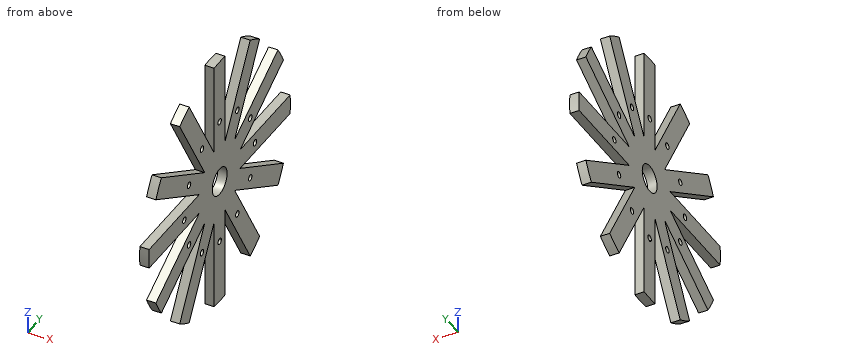
```python
from build123d import *

# Parameters (mm, degrees)
SKETCH1_W           = 450
SKETCH1_H           = 450
BOSS_EXTRUDE1_DEPTH = 5
BOSS_EXTRUDE2_DEPTH = 7.48
BOSS_EXTRUDE3_DEPTH = 7.48
SKETCH6_W           = 450
SKETCH6_H           = 450
CUT_EXTRUDE1_DEPTH  = 5
SKETCH7_R           = 11
SKETCH7_R_2         = 2.5
CUT_EXTRUDE2_DEPTH  = 10
SKETCH8_R           = 209.3091
SKETCH8_R_2         = 104.5891
CUT_EXTRUDE3_DEPTH  = 10
BOSS_EXTRUDE4_DEPTH = 7.48
SKETCH11_R          = 2.5
CUT_EXTRUDE5_DEPTH  = 10
SKETCH12_R          = 20.73675099
SKETCH12_R_2        = 11
BOSS_EXTRUDE5_DEPTH = 7.48


# Read off the part's stored shape, not the designer's step: Boss-Extrude2
with BuildPart() as part:
    # Sketch1 → Boss-Extrude1 (new body)
    with BuildSketch(Plane(origin=(0, 0, 0), x_dir=(0, 0, -1), z_dir=(1, 0, 0))):
        Rectangle(SKETCH1_W, SKETCH1_H)
    extrude(amount=BOSS_EXTRUDE1_DEPTH)

    # Boss-Extrude2 outline → Boss-Extrude2 (add)
    with BuildSketch(Plane(origin=(5, 0, 0), x_dir=(0, 0, -1), z_dir=(1, 0, 0))):
        with BuildLine():
            Line((-164.971757583, 8.09), (-209.152698388, 8.09))
            ThreePointArc((-209.152698388, 8.09), (-209.3091, 0), (-209.152698388, -8.09))
            Line((-209.152698388, -8.09), (-164.971757583, -8.09))
            ThreePointArc((-164.971757583, -8.09), (-116.792827049, -116.792827049), (-8.09, -164.971757583))
            Line((-8.09, -164.971757583), (-8.09, -209.152698388))
            ThreePointArc((-8.09, -209.152698388), (0, -209.3091), (8.09, -209.152698388))
            Line((8.09, -209.152698388), (8.09, -164.971757583))
            ThreePointArc((8.09, -164.971757583), (116.792827049, -116.792827049), (164.971757583, -8.09))
            Line((164.971757583, -8.09), (209.152698388, -8.09))
            ThreePointArc((209.152698388, -8.09), (209.3091, 0), (209.152698388, 8.09))
            Line((209.152698388, 8.09), (164.971757583, 8.09))
            ThreePointArc((164.971757583, 8.09), (116.792827049, 116.792827049), (8.09, 164.971757583))
            Line((8.09, 164.971757583), (8.09, 209.152698388))
            ThreePointArc((8.09, 209.152698388), (0, 209.3091), (-8.09, 209.152698388))
            Line((-8.09, 209.152698388), (-8.09, 164.971757583))
            ThreePointArc((-8.09, 164.971757583), (-116.792827049, 116.792827049), (-164.971757583, 8.09))
        make_face()
        with BuildLine():
            Line((148.770198629, 8.09), (104.538333308, 8.09))
            ThreePointArc((104.538333308, 8.09), (104.8509, 0), (104.538333308, -8.09))
            Line((104.538333308, -8.09), (148.770198629, -8.09))
            ThreePointArc((148.770198629, -8.09), (105.351839329, -105.351839329), (8.09, -148.770198629))
            Line((8.09, -148.770198629), (8.09, -104.538333308))
            ThreePointArc((8.09, -104.538333308), (0, -104.8509), (-8.09, -104.538333308))
            Line((-8.09, -104.538333308), (-8.09, -148.770198629))
            ThreePointArc((-8.09, -148.770198629), (-105.351839329, -105.351839329), (-148.770198629, -8.09))
            Line((-148.770198629, -8.09), (-104.538333308, -8.09))
            ThreePointArc((-104.538333308, -8.09), (-104.8509, 0), (-104.538333308, 8.09))
            Line((-104.538333308, 8.09), (-148.770198629, 8.09))
            ThreePointArc((-148.770198629, 8.09), (-105.351839329, 105.351839329), (-8.09, 148.770198629))
            Line((-8.09, 148.770198629), (-8.09, 104.538333308))
            ThreePointArc((-8.09, 104.538333308), (0, 104.8509), (8.09, 104.538333308))
            Line((8.09, 104.538333308), (8.09, 148.770198629))
            ThreePointArc((8.09, 148.770198629), (105.351839329, 105.351839329), (148.770198629, 8.09))
        make_face(mode=Mode.SUBTRACT)
    extrude(amount=BOSS_EXTRUDE2_DEPTH)

    # Sketch5 → Boss-Extrude3 (add)
    with BuildSketch(Plane(origin=(5, 0, 0), x_dir=(0, 0, -1), z_dir=(1, 0, 0))):
        with BuildLine():
            Line((-19.319547743, 8.09), (-104.275748565, 8.09))
            ThreePointArc((-104.275748565, 8.09), (-104.5891, 0), (-104.275748565, -8.09))
            Line((-104.275748565, -8.09), (-19.319547743, -8.09))
            ThreePointArc((-19.319547743, -8.09), (0, -20.945), (19.319547743, -8.09))
            Line((19.319547743, -8.09), (104.275748565, -8.09))
            ThreePointArc((104.275748565, -8.09), (104.5891, 0), (104.275748565, 8.09))
            Line((104.275748565, 8.09), (19.319547743, 8.09))
            ThreePointArc((19.319547743, 8.09), (0, 20.945), (-19.319547743, 8.09))
        make_face()
    extrude(amount=BOSS_EXTRUDE3_DEPTH)

    # Sketch6 → Cut-Extrude1 (cut)
    with BuildSketch(Plane.ZY):
        Rectangle(SKETCH6_W, SKETCH6_H)
    extrude(amount=-CUT_EXTRUDE1_DEPTH, mode=Mode.SUBTRACT)


with BuildPart() as cut_extrude1_piece_1:
    # of the separate pieces the step leaves, piece 1, a body of its own (cut_extrude1_pieces)
    add(part.part.solids().sort_by_distance((5, 209.152698388, 8.09))[0])


with BuildPart() as cut_extrude1_piece_2:
    # of the separate pieces the step leaves, piece 2, a body of its own (cut_extrude1_pieces)
    add(part.part.solids().sort_by_distance((5, 8.09, -104.275748565))[0])


with BuildPart() as cut_extrude2_tool:
    # Sketch7 → Cut-Extrude2 (new body)
    with BuildSketch(Plane(origin=(12.48, 0, 0), x_dir=(0, 0, -1), z_dir=(1, 0, 0))):
        Circle(SKETCH7_R)
        with Locations((-183.1891, 0)):
            Circle(SKETCH7_R_2)
        with Locations((-130.9659, 0)):
            Circle(SKETCH7_R_2)
        with Locations((0, -183.1891)):
            Circle(SKETCH7_R_2)
        with Locations((0, -130.9659)):
            Circle(SKETCH7_R_2)
        with Locations((183.1891, 0)):
            Circle(SKETCH7_R_2)
        with Locations((52.3, 0)):
            Circle(SKETCH7_R_2)
        with Locations((-52.295, 0)):
            Circle(SKETCH7_R_2)
        with Locations((0, 183.1891)):
            Circle(SKETCH7_R_2)
        with Locations((0, 130.9659)):
            Circle(SKETCH7_R_2)
        with BuildLine():
            Line((-3, 13.8), (-3, 10.583005244))
            ThreePointArc((-3, 10.583005244), (0, 11), (3, 10.583005244))
            Line((3, 10.583005244), (3, 13.8))
            Line((3, 13.8), (-3, 13.8))
        make_face()
        with BuildLine():
            ThreePointArc((3, -10.583005244), (0, -11), (-3, -10.583005244))
            Line((-3, -10.583005244), (-3, -13.8))
            Line((-3, -13.8), (3, -13.8))
            Line((3, -13.8), (3, -10.583005244))
        make_face()
        with Locations((130.9659, 0)):
            Circle(SKETCH7_R_2)
    extrude(amount=-CUT_EXTRUDE2_DEPTH)


with BuildPart() as cut_extrude1_piece_1_1:
    add(cut_extrude1_piece_1.part)

    # Cut-Extrude2: cut by cut_extrude2_tool
    add(cut_extrude2_tool.part, mode=Mode.SUBTRACT)

    # Sketch8 → Cut-Extrude3 (cut)
    with BuildSketch(Plane(origin=(12.48, 0, 0), x_dir=(0, 0, -1), z_dir=(1, 0, 0))):
        Circle(SKETCH8_R)
        Circle(SKETCH8_R_2, mode=Mode.SUBTRACT)
    extrude(amount=-CUT_EXTRUDE3_DEPTH, mode=Mode.SUBTRACT)


with BuildPart() as cut_extrude1_piece_2_1:
    add(cut_extrude1_piece_2.part)

    # Cut-Extrude2: cut by cut_extrude2_tool
    add(cut_extrude2_tool.part, mode=Mode.SUBTRACT)

    # Sketch9 → Boss-Extrude4 (add)
    with BuildSketch(Plane(origin=(12.48, 0, 0), x_dir=(0, 0, -1), z_dir=(1, 0, 0))):
        with BuildLine():
            Line((-94.350447256, 45.131728766), (-30.192291033, 8.09))
            Line((-30.192291033, 8.09), (-19.319547743, 8.09))
            ThreePointArc((-19.319547743, 8.09), (0, 20.945), (19.319547743, 8.09))
            Line((19.319547743, 8.09), (30.192291033, 8.09))
            Line((30.192291033, 8.09), (94.350447256, 45.131728766))
            ThreePointArc((94.350447256, 45.131728766), (90.576817559, 52.29455), (86.260447256, 59.144019799))
            Line((86.260447256, 59.144019799), (22.102291033, 22.102291033))
            Line((22.102291033, 22.102291033), (59.144019799, 86.260447256))
            ThreePointArc((59.144019799, 86.260447256), (52.29455, 90.576817559), (45.131728766, 94.350447256))
            Line((45.131728766, 94.350447256), (8.09, 30.192291033))
            Line((8.09, 30.192291033), (8.09, 104.275748565))
            ThreePointArc((8.09, 104.275748565), (0, 104.5891), (-8.09, 104.275748565))
            Line((-8.09, 104.275748565), (-8.09, 30.192291033))
            Line((-8.09, 30.192291033), (-45.131728766, 94.350447256))
            ThreePointArc((-45.131728766, 94.350447256), (-52.29455, 90.576817559), (-59.144019799, 86.260447256))
            Line((-59.144019799, 86.260447256), (-22.102291033, 22.102291033))
            Line((-22.102291033, 22.102291033), (-86.260447256, 59.144019799))
            ThreePointArc((-86.260447256, 59.144019799), (-90.576817559, 52.29455), (-94.350447256, 45.131728766))
        make_face()
        with BuildLine():
            ThreePointArc((19.319547743, -8.09), (0, -20.945), (-19.319547743, -8.09))
            Line((-19.319547743, -8.09), (-30.192291033, -8.09))
            Line((-30.192291033, -8.09), (-94.350447256, -45.131728766))
            ThreePointArc((-94.350447256, -45.131728766), (-90.576817559, -52.29455), (-86.260447256, -59.144019799))
            Line((-86.260447256, -59.144019799), (-22.102291033, -22.102291033))
            Line((-22.102291033, -22.102291033), (-59.144019799, -86.260447256))
            ThreePointArc((-59.144019799, -86.260447256), (-52.29455, -90.576817559), (-45.131728766, -94.350447256))
            Line((-45.131728766, -94.350447256), (-8.09, -30.192291033))
            Line((-8.09, -30.192291033), (-8.09, -104.275748565))
            ThreePointArc((-8.09, -104.275748565), (0, -104.5891), (8.09, -104.275748565))
            Line((8.09, -104.275748565), (8.09, -30.192291033))
            Line((8.09, -30.192291033), (45.131728766, -94.350447256))
            ThreePointArc((45.131728766, -94.350447256), (52.29455, -90.576817559), (59.144019799, -86.260447256))
            Line((59.144019799, -86.260447256), (22.102291033, -22.102291033))
            Line((22.102291033, -22.102291033), (86.260447256, -59.144019799))
            ThreePointArc((86.260447256, -59.144019799), (90.576817559, -52.29455), (94.350447256, -45.131728766))
            Line((94.350447256, -45.131728766), (30.192291033, -8.09))
            Line((30.192291033, -8.09), (19.319547743, -8.09))
        make_face()
    extrude(amount=-BOSS_EXTRUDE4_DEPTH)

    # Sketch11 → Cut-Extrude5 (cut)
    with BuildSketch(Plane(origin=(12.48, 0, 0), x_dir=(0, 0, -1), z_dir=(1, 0, 0))):
        with Locations((-52.295, 0)):
            Circle(SKETCH11_R)
        with Locations((-45.288798491, 26.1475)):
            Circle(SKETCH11_R)
        with Locations((-26.1475, 45.288798491)):
            Circle(SKETCH11_R)
        with Locations((0, 52.295)):
            Circle(SKETCH11_R)
        with Locations((26.1475, 45.288798491)):
            Circle(SKETCH11_R)
        with Locations((45.288798491, 26.1475)):
            Circle(SKETCH11_R)
        with Locations((52.295, 0)):
            Circle(SKETCH11_R)
        with Locations((45.288798491, -26.1475)):
            Circle(SKETCH11_R)
        with Locations((26.1475, -45.288798491)):
            Circle(SKETCH11_R)
        with Locations((0, -52.295)):
            Circle(SKETCH11_R)
        with Locations((-26.1475, -45.288798491)):
            Circle(SKETCH11_R)
        with Locations((-45.288798491, -26.1475)):
            Circle(SKETCH11_R)
    extrude(amount=-CUT_EXTRUDE5_DEPTH, mode=Mode.SUBTRACT)

    # Sketch12 → Boss-Extrude5 (add)
    with BuildSketch(Plane(origin=(12.48, 0, 0), x_dir=(0, 0, -1), z_dir=(1, 0, 0))):
        Circle(SKETCH12_R)
        Circle(SKETCH12_R_2, mode=Mode.SUBTRACT)
    extrude(amount=-BOSS_EXTRUDE5_DEPTH)


solid = cut_extrude1_piece_2_1.part
```
Input: part model. Units: mm. Frame: model coordinates. Round coordinates to 2 decimals unless told otherwise and drop trailing zeros. Write each loop counter-clockwise with the first axis right and the second up, starting at its lowest first coordinate (ties: lowest second). Pieces come first, ordered by that corner, then holes. Notation, with made-up numbers: M 86.5,85 L 121.5,85 A10 cw 121.5,89 Z; hole C -28.75,43.5 d6. An arc over 180 degrees is marked long. Write each question's results on one line, items separated by ' | '.
Q1. Section query C-C (x = 11). State how many separate pieces and enclosed holes the cut face has, and give its area (3 significant figures).
Results:
separate pieces: 1 | enclosed holes: 13 | area: 16,700 mm^2
Q2. Pin query (flat end, axial travel): P1, Ø4, axis at x = 7, y = 7, coming from the +Z side; P2, Ø2, axis at x = 7, z = 72, coming from the +Y side. Return the tip coordinate at first contact, or that it passes through.
Results:
P1: stops at z = 104.47 | P2: stops at y = 51.49
Q3. Section query A-A (z = 0). Return loops of the section in (x, y) (3 decimals).
Results:
outline: M 5,-104.589 L 12.48,-104.589 L 12.48,-54.795 L 5,-54.795 Z; M 5,-49.795 L 12.48,-49.795 L 12.48,-11 L 5,-11 Z; M 5,11 L 12.48,11 L 12.48,49.795 L 5,49.795 Z; M 5,54.795 L 12.48,54.795 L 12.48,104.589 L 5,104.589 Z
Q4. Line query: line 1 along Y through (x, z) = (12, 83); line 2 along Z through (x, y) = (9.75, -48.5); line 3 along Z through (x, y) = (11, -75). Output: solid intervals per line, ascending.
Results:
line 1: y = -57.26 to -38.58, -8.09 to 8.09, 38.58 to 57.26 | line 2: z = -92.66 to -67.82, -37.34 to -18.66, -8.09 to 8.09, 18.66 to 37.34, 67.82 to 92.66 | line 3: z = -52.64 to -33.96, -8.09 to 8.09, 33.96 to 52.64
Q5. Section query B-B (y = 0). Return loops of the section in (x, z) (3 decimals).
Results:
outline: M 5,-104.589 L 12.48,-104.589 L 12.48,-54.8 L 5,-54.8 Z; M 5,-49.795 L 12.48,-49.795 L 12.48,-11 L 5,-11 Z; M 5,11 L 12.48,11 L 12.48,49.795 L 5,49.795 Z; M 5,54.795 L 12.48,54.795 L 12.48,104.589 L 5,104.589 Z
